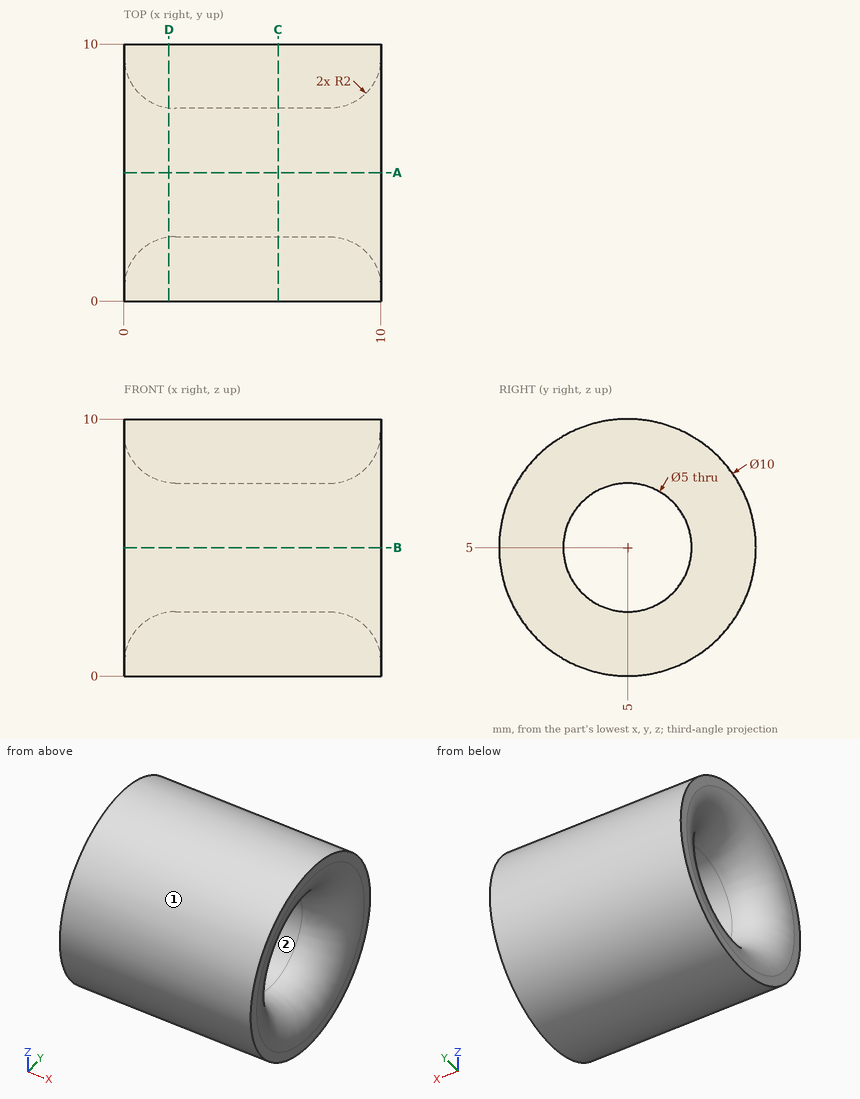
Design review of the part shown in the three views and the two pictorial views. Dimensions are in mm from the part's minimum x, y and z. Coordinates: 2 decimals unless noted, no trailing zeros. Write each loop counter-clockwise with the first axis right and the second up, starting at its lowest first coordinate (ties: lowest second). Pieces come first, ordered by that corner, then holes. Notation, with made-up numbers: (-29, 42) - (29, 42) arc R15 ccw to (29, 67) - close; hole circle Ø11 at (82, 43.5). An arc over 180 degrees is marked (long way). Write item = value, one per line.
(1) For line 1 (Z direction, x = 5, y = 5); line 2 (Y direction, x = 4, z = 3.5); line 3 (Y direction, x = 4.25, z = 3.25), list the stretches that pass through material, from the lowest coordinate up. Write a range as [from, to].
Result sheet:
line_1 = [0, 2.5], [7.5, 10]
line_2 = [0.23, 3], [7, 9.77]
line_3 = [0.32, 3.21], [6.79, 9.68]
(2) For P1, Ø1, axis at x = 4, z = 1, coming from the -Y side; P2, Ø4, axis at y = 1.5, z = 6, coming from the +X side; P3, Ø2, axis at x = 6.5, y = 8, coming from the -Z side; P4, Ø1.5, axis at y = 7, z = 6.5, coming from the -X side, all flat-tipped, find the tip position at first contact; note any pin that passes through.
Result sheet:
P1 = 1.43
P2 = 10
P3 = 0.42
P4 = 0.44
(3) Consider section A-A, the plane y = 5. Give the boundary of the cut face in (x, z).
Result sheet:
outline = (0, 0) - (10, 0) - (10, 0.5) arc R2 ccw to (8, 2.5) - (2, 2.5) arc R2 ccw to (0, 0.5) - close; (0, 9.5) arc R2 ccw to (2, 7.5) - (8, 7.5) arc R2 ccw to (10, 9.5) - (10, 10) - (0, 10) - close
(4) Mouldability with a two-part tool opening along Y and no side actions: class the marked faces 1 and 2 as pulls with the +Y half, pulls with the -Y half, needs draft (parallel to the pull), parting line crosses it, or undercut.
Result sheet:
face_1 = parting line crosses it
face_2 = undercut
(5) Consider section C-C, the plane x = 6. Give the boundary of the cut face in (y, z).
Result sheet:
outline = circle Ø10 at (5, 5); hole circle Ø5 at (5, 5)
(6) Consider section D-D, the plane x = 1.75. Give the boundary of the cut face in (y, z), then the cut area to 3 significant figures.
Result sheet:
outline = circle Ø10 at (5, 5); hole circle Ø5.03 at (5, 5)
area = 58.7 mm^2
